Can you work these out from the model? Positions are in its coordinate system, mm. Face numbers are marked on the shaded views. Coordinates: 2 decimals unless noted, no trailing zeros. Order: outer loops, then holes, each group sorted by start corner. A loop starts at its lowest first (then second) coordinate and runs counter-clockwise, first axis right, second up. Notation, with made-up numbers: (33.25, 86) -> (44.25, 86) arc R23 cw to (44.25, 107) -> close; hole circle Ø10 at (-4.75, 78). An arc over 180 degrees is marked (long way). Return JSON: item names as keys, results as strings. Group by question number.
1) Thinking about a two-plate mould opening in X: for the marked faces 1, 2 and 3, which applies, +X half, -X half, draft (parallel to the pull), parting line (faces both ways), or undercut?
2) If we section it at B-B, the plane x = 0: Please give me the cut outline in (y, z) (3 decimals).
3) If we section it at A-A, the plane z = 0: Please give me the cut outline in (x, y) (3 decimals).
4) If we section it at C-C, the plane x = 44.5: Please give me the cut outline in (y, z) (3 decimals), then the cut area to 3 significant figures.
5) For pin 1 (6 mm diameter, centred on x = -27.5, z = -41, fed in from +Y) (3 decimals); pin 2 (8 mm diameter, centred on x = 40.5, z = -21.5, fed in from +Y) (3 decimals); pin 3 (4 mm diameter, centred on x = -10, y = 5.5, fed in from -Z); pin 4 (5 mm diameter, centred on x = -27.5, z = -27, fed in from -Y), each with a flat end and sliding along its axis, tell me the tip position at first contact or that it passes through.
6) If I drill on probe 1 along X at (y, z) = (3.8, 0) (3 decimals); probe 2 along X at (y, z) = (3.75, -2.5); probe 3 along Z at (x, y) = (1.5, 1.75), over which ranges is the centre line in solid material (lowest first)? Write a range as from..to.
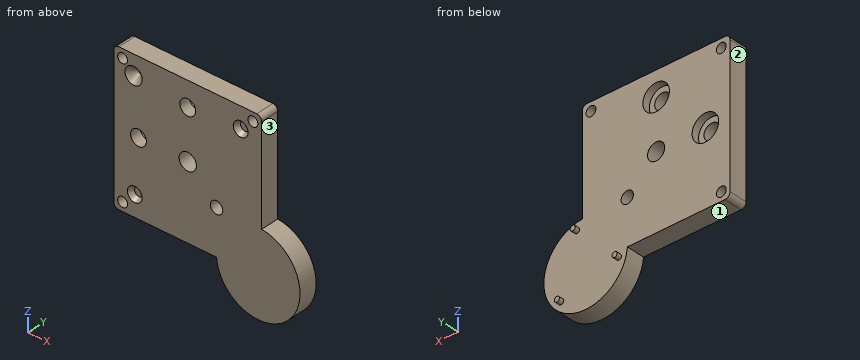
from build123d import *

# Parameters (mm, degrees)
SKETCH1_W                    = 76.2
SKETCH1_H                    = 76.2
BOSS_EXTRUDE1_DEPTH          = 9.525
SKETCH6_R                    = 3.81
CUT_EXTRUDE2_DEPTH           = 2.54
CUT_EXTRUDE2_DRAFT           = 30
CUT_EXTRUDE2_PROFILE_2_DEPTH = 2.54
CUT_EXTRUDE2_PROFILE_2_DRAFT = 30
CUT_EXTRUDE4_REACH           = 56.717
SKETCH12_R                   = 4.064
SKETCH13_R                   = 6.858
CUT_EXTRUDE7_DEPTH           = 3.81
SKETCH7_R                    = 4.445
CUT_EXTRUDE8_DEPTH           = 3.81
CUT_EXTRUDE8_TAPER           = 45
CUT_EXTRUDE9_REACH           = 56.717
SKETCH15_R                   = 4.445
FILLET1_R                    = 2.54
SKETCH17_R                   = 21.59
BOSS_EXTRUDE2_DEPTH          = 9.525
SKETCH18_R                   = 1.3335
BOSS_EXTRUDE3_DEPTH          = 2.54
CUT_EXTRUDE10_REACH          = 84.437
SKETCH20_R                   = 2.54
SKETCH20_R_2                 = 3.175


with BuildPart() as part:
    # Sketch1 → Boss-Extrude1 (new body)
    with BuildSketch(Plane(origin=(0, 0, 0), x_dir=(1, 0, 0), z_dir=(0, 1, 0))):
        Rectangle(SKETCH1_W, SKETCH1_H)
    extrude(amount=BOSS_EXTRUDE1_DEPTH)


with BuildPart() as cut_extrude2_tool:
    # Sketch6 → Cut-Extrude2 (with draft: the straight prism first)
    with BuildSketch(Plane(origin=(0, 0, 0), x_dir=(1, 0, 0), z_dir=(0, 1, 0))):
        with Locations((-27.323692655, 27.323692655)):
            Circle(SKETCH6_R)
    extrude(amount=CUT_EXTRUDE2_DEPTH)
    # Cut-Extrude2: the draft: its side faces are tilted about the plane it starts from
    cut_extrude2_sides = [cut_extrude2_tool.faces().sort_by_distance(p)[0] for p in [
        (-31.133692655, 1.27, -27.323692655),
    ]]
    draft(cut_extrude2_sides, Plane(origin=(0, 0, 0), x_dir=(1, 0, 0), z_dir=(0, 1, 0)), CUT_EXTRUDE2_DRAFT)


with BuildPart() as part_1:
    add(part.part)

    # Cut-Extrude2: cut by cut_extrude2_tool
    add(cut_extrude2_tool.part, mode=Mode.SUBTRACT)


with BuildPart() as cut_extrude2_profile_2_tool:
    # Sketch6 → Cut-Extrude2 profile 2 (with draft: the straight prism first)
    with BuildSketch(Plane(origin=(0, 0, 0), x_dir=(1, 0, 0), z_dir=(0, 1, 0))):
        with Locations((27.323692655, -27.323692655)):
            Circle(SKETCH6_R)
    extrude(amount=CUT_EXTRUDE2_PROFILE_2_DEPTH)
    # Cut-Extrude2 profile 2: the draft: its side faces are tilted about the plane it starts from
    cut_extrude2_profile_2_sides = [cut_extrude2_profile_2_tool.faces().sort_by_distance(p)[0] for p in [
        (23.513692655, 1.27, 27.323692655),
    ]]
    draft(cut_extrude2_profile_2_sides, Plane(origin=(0, 0, 0), x_dir=(1, 0, 0), z_dir=(0, 1, 0)), CUT_EXTRUDE2_PROFILE_2_DRAFT)


with BuildPart() as part_2:
    add(part_1.part)

    # Cut-Extrude2 profile 2: cut by cut_extrude2_profile_2_tool
    add(cut_extrude2_profile_2_tool.part, mode=Mode.SUBTRACT)

    # Sketch12 → Cut-Extrude4 (cut, up to next)
    with BuildSketch(Plane(origin=(0, 9.525, 0), x_dir=(1, 0, 0), z_dir=(0, 1, 0)), mode=Mode.PRIVATE) as cut_extrude4_sk1:
        with Locations(Location((-25.4, 0, 0), (0, 0, 270))):
            Circle(SKETCH12_R)
    cut_extrude4_tool1 = extrude(cut_extrude4_sk1.sketch, amount=-CUT_EXTRUDE4_REACH, mode=Mode.PRIVATE) & part_2.part
    # Sketch12 → Cut-Extrude4 (cut, up to next)
    with BuildSketch(Plane(origin=(0, 9.525, 0), x_dir=(1, 0, 0), z_dir=(0, 1, 0)), mode=Mode.PRIVATE) as cut_extrude4_sk2:
        with Locations(Location((0, -25.4, 0), (0, 0, 270))):
            Circle(SKETCH12_R)
    cut_extrude4_tool2 = extrude(cut_extrude4_sk2.sketch, amount=-CUT_EXTRUDE4_REACH, mode=Mode.PRIVATE) & part_2.part
    add(cut_extrude4_tool1.solids().sort_by_distance((-25.4, 9.525, 0))[0], mode=Mode.SUBTRACT)
    add(cut_extrude4_tool2.solids().sort_by_distance((0, 9.525, 25.4))[0], mode=Mode.SUBTRACT)

    # Sketch13 → Cut-Extrude7 (cut)
    with BuildSketch(Plane.XZ.offset(-9.525)):
        with Locations(Location((-25.4, 0, 0), (0, 0, 90))):
            Circle(SKETCH13_R)
        with Locations(Location((0, 25.4, 0), (0, 0, 90))):
            Circle(SKETCH13_R)
    extrude(amount=CUT_EXTRUDE7_DEPTH, mode=Mode.SUBTRACT)

    # Sketch7 → Cut-Extrude8 (cut)
    with BuildSketch(Plane(origin=(0, 0, 0), x_dir=(1, 0, 0), z_dir=(0, 1, 0))):
        with Locations((-27.94, -27.94)):
            Circle(SKETCH7_R)
    extrude(amount=CUT_EXTRUDE8_DEPTH, taper=CUT_EXTRUDE8_TAPER, mode=Mode.SUBTRACT)

    # Sketch15 → Cut-Extrude9 (cut, up to next)
    with BuildSketch(Plane(origin=(0, 9.525, 0), x_dir=(1, 0, 0), z_dir=(0, 1, 0)), mode=Mode.PRIVATE) as cut_extrude9_sk1:
        with Locations(Location((0, 0, 0), (0, 0, 270))):
            Circle(SKETCH15_R)
    cut_extrude9_tool1 = extrude(cut_extrude9_sk1.sketch, amount=-CUT_EXTRUDE9_REACH, mode=Mode.PRIVATE) & part_2.part
    add(cut_extrude9_tool1.solids().sort_by_distance((0, 9.525, 0))[0], mode=Mode.SUBTRACT)

    # Fillet1
    fillet1_edges = [part_2.edges().sort_by_distance(p)[0] for p in [
        (38.1, 4.7625, 38.1),
        (-38.1, 4.7625, 38.1),
        (-38.1, 4.7625, -38.1),
        (38.1, 4.7625, -38.1),
    ]]
    fillet(fillet1_edges, radius=FILLET1_R)

    # Sketch17 → Boss-Extrude2 (add)
    with BuildSketch(Plane(origin=(0, 9.525, 0), x_dir=(1, 0, 0), z_dir=(0, 1, 0))):
        with Locations((36.311274722, 36.311274722)):
            Circle(SKETCH17_R)
    extrude(amount=-BOSS_EXTRUDE2_DEPTH)

    # Sketch18 → Boss-Extrude3 (add)
    with BuildSketch(Plane(origin=(0, 9.525, 0), x_dir=(1, 0, 0), z_dir=(0, 1, 0))):
        with Locations(Location((19.166305808, 41.020673934, 0), (0, 0, 270))):
            Circle(SKETCH18_R)
        with Locations(Location((48.962218533, 48.804553742, 0), (0, 0, 270))):
            Circle(SKETCH18_R)
        with Locations(Location((40.805299824, 19.108596489, 0), (0, 0, 270))):
            Circle(SKETCH18_R)
    extrude(amount=BOSS_EXTRUDE3_DEPTH)

    # Sketch20 → Cut-Extrude10 (cut, up to next)
    with BuildSketch(Plane(origin=(0, 9.525, 0), x_dir=(1, 0, 0), z_dir=(0, 1, 0)), mode=Mode.PRIVATE) as cut_extrude10_sk1:
        with Locations(Location((-33.609871939, -33.609871939, 0), (0, 0, 270))):
            Circle(SKETCH20_R)
    cut_extrude10_tool1 = extrude(cut_extrude10_sk1.sketch, amount=-CUT_EXTRUDE10_REACH, mode=Mode.PRIVATE) & part_2.part
    # Sketch20 → Cut-Extrude10 (cut, up to next)
    with BuildSketch(Plane(origin=(0, 9.525, 0), x_dir=(1, 0, 0), z_dir=(0, 1, 0)), mode=Mode.PRIVATE) as cut_extrude10_sk2:
        with Locations(Location((33.609871939, -33.609871939, 0), (0, 0, 270))):
            Circle(SKETCH20_R)
    cut_extrude10_tool2 = extrude(cut_extrude10_sk2.sketch, amount=-CUT_EXTRUDE10_REACH, mode=Mode.PRIVATE) & part_2.part
    # Sketch20 → Cut-Extrude10 (cut, up to next)
    with BuildSketch(Plane(origin=(0, 9.525, 0), x_dir=(1, 0, 0), z_dir=(0, 1, 0)), mode=Mode.PRIVATE) as cut_extrude10_sk3:
        with Locations(Location((-33.609871939, 33.609871939, 0), (0, 0, 270))):
            Circle(SKETCH20_R)
    cut_extrude10_tool3 = extrude(cut_extrude10_sk3.sketch, amount=-CUT_EXTRUDE10_REACH, mode=Mode.PRIVATE) & part_2.part
    # Sketch20 → Cut-Extrude10 (cut, up to next)
    with BuildSketch(Plane(origin=(0, 9.525, 0), x_dir=(1, 0, 0), z_dir=(0, 1, 0)), mode=Mode.PRIVATE) as cut_extrude10_sk4:
        with Locations(Location((14.883511114, 14.883511114, 0), (0, 0, 270))):
            Circle(SKETCH20_R_2)
    cut_extrude10_tool4 = extrude(cut_extrude10_sk4.sketch, amount=-CUT_EXTRUDE10_REACH, mode=Mode.PRIVATE) & part_2.part
    add(cut_extrude10_tool1.solids().sort_by_distance((-33.609872, 9.525, 33.609872))[0], mode=Mode.SUBTRACT)
    add(cut_extrude10_tool2.solids().sort_by_distance((33.609872, 9.525, 33.609872))[0], mode=Mode.SUBTRACT)
    add(cut_extrude10_tool3.solids().sort_by_distance((-33.609872, 9.525, -33.609872))[0], mode=Mode.SUBTRACT)
    add(cut_extrude10_tool4.solids().sort_by_distance((14.883511, 9.525, -14.883511))[0], mode=Mode.SUBTRACT)


solid = part_2.part
Result sheet:
{
 "1": {"face 1": "draft", "face 2": "-X half", "face 3": "+X half"},
 "2": {"outline": "(0, -38.1) -> (9.525, -38.1) -> (9.525, -4.445) -> (0, -4.445) -> close; (0, 4.445) -> (9.525, 4.445) -> (9.525, 18.542) -> (5.715, 18.542) -> (5.715, 21.336) -> (0, 21.336) -> close; (0, 29.464) -> (5.715, 29.464) -> (5.715, 32.258) -> (9.525, 32.258) -> (9.525, 38.1) -> (0, 38.1) -> close"},
 "3": {"outline": "(-38.1, 0) -> (-29.464, 0) -> (-29.464, 5.715) -> (-32.258, 5.715) -> (-32.258, 9.525) -> (-38.1, 9.525) -> close; (-21.336, 0) -> (-4.445, 0) -> (-4.445, 9.525) -> (-18.542, 9.525) -> (-18.542, 5.715) -> (-21.336, 5.715) -> close; (4.445, 0) -> (38.1, 0) -> (38.1, 9.525) -> (4.445, 9.525) -> close"},
 "4": {"outline": "(0, -56.288) -> (9.525, -56.288) -> (9.525, -16.334) -> (0, -16.334) -> close", "area": "381 mm2"},
 "5": {"pin 1": "stops at y = 9.525", "pin 2": "stops at y = 12.065", "pin 3": "stops at z = -38.1", "pin 4": "stops at y = 1.63"},
 "6": {"probe 1": "x = -38.1..-29.464, -21.336..-4.445, 4.445..38.1", "probe 2": "x = -38.1..-28.6, -22.2..-3.68, 3.68..38.1", "probe 3": "z = -38.1..-4.18, 4.18..21.62, 29.18..38.1"}
}
